Read the model definition and answer for the solid it produces. Units are mm, in the model's axes. A direction names the side the tool comes from. Give positions to 0.01 mm unless a question says otherwise; leave off trailing zeros. Loops run counter-clockwise (first coordinate to the right, second up) from the corner with the lowest first, then second, coordinate; pieces in that order, holes last. Notation, with made-up numbers: M -3,-15 L 4,-15 A33 ccw 4,18 Z; hole C -33,-38 d8. An arc over 180 degrees is marked long. Return JSON: item names as keys, results as strings. Group by question number.
```python
from build123d import *

# Parameters (mm, degrees)
F0_R     = 41.275
F1_DEPTH = 101.6
F2_W     = 82.747999
F2_H     = 29.89918
F3_DEPTH = 36.83
F4_R     = 40.005
F5_DEPTH = 98.044
F6_R     = 41.275
F7_DEPTH = 6.35


with BuildPart() as f1:
    # F0 (on Front) → F1 (new body, symmetric)
    with BuildSketch(Plane.XZ):
        Circle(F0_R)
    extrude(amount=F1_DEPTH, both=True)

    # F2 (on Top) → F3 (cut, symmetric)
    with BuildSketch(Plane.XY):
        with Locations((-0.162097, -78.476146)):
            Rectangle(F2_W, F2_H)
    extrude(amount=F3_DEPTH, both=True, mode=Mode.SUBTRACT)

    # F4 (on Front) → F5 (cut, symmetric)
    with BuildSketch(Plane.XZ):
        Circle(F4_R)
    extrude(amount=F5_DEPTH, both=True, mode=Mode.SUBTRACT)

    # F6 (on face) → F7 (cut, symmetric)
    with BuildSketch(Plane(origin=(0, 101.6, 0), x_dir=(-1, 0, 0), z_dir=(0, 1, 0))):
        Circle(F6_R)
    extrude(amount=F7_DEPTH, both=True, mode=Mode.SUBTRACT)


solid = f1.part
```
1. Straight lines are drawn through the part: line 1 along Z through (x, y) = (0, -51) (3 decimals); line 2 along X through (y, z) = (-54, 0.5); line 3 along Y through (x, z) = (33, 24). For each, find the intervals that lie inside material, in ascending order.
2. Find section B-B (x = -33). Write down the section's boundary in (y, z), and give its area (3 significant figures).
3. Find section D-D (x = 0). Write down the section's boundary in (y, z) (3 decimals).
4. The mould has two halves that part along Y. Classify faces 1 (the flat face through (-1, -101.6, 1)), 2 (the flat face through (-1, -98.044, 1)), 3 (the flat face through (-41, -93.426, 0)): +Y half, -Y half, draft (parallel to the pull), parting line (faces both ways), or undercut.
5. Find section C-C (z = 23.5). Write down the section's boundary in (x, y), and give its area (3 significant figures).
6. Flat-ended cylindrical pins translate along their axes: P1, Ø1.5, axis at y = -34, z = 24.5, coming from the +X side; P2, Ø1.5, axis at y = 72.5, z = 7, coming from the -X side; P3, Ø4, axis at x = -13.5, z = -26, coming from the +Y side. Find the tip coordinate at first contact, or state that the pin passes through.
7. For faces 4 (the cylindrical face through (-39.966, 18.727, 1.759)), 5 (the cylindrical face through (-41.235, 17.319, 1.815)), determine the directions among +Z, -Z, +X, -X, +Y, -Y from which every point of the face is accessible in a straight line to the end or side of a thin tool.
8. Find section A-A (z = 0). Write down the section's boundary in (x, y) (3 decimals), and give its area (3 significant figures).
Result:
{
 "1": {"line 1": "z = -41.275 to -40.005, 40.005 to 41.275", "line 2": "x = -41.27 to -40, 40 to 41.27", "line 3": "y = -101.6 to -93.43, -63.53 to 95.25"},
 "2": {"outline": "M -101.6,-24.79 L -93.43,-24.79 L -93.43,-22.61 L -98.04,-22.61 L -98.04,22.61 L -93.43,22.61 L -93.43,24.79 L -101.6,24.79 Z; M -63.53,-24.79 L 95.25,-24.79 L 95.25,-22.61 L -63.53,-22.61 Z; M -63.53,22.61 L 95.25,22.61 L 95.25,24.79 L -63.53,24.79 Z", "area": "888 mm2"},
 "3": {"outline": "M -101.6,-41.275 L 95.25,-41.275 L 95.25,-40.005 L -98.044,-40.005 L -98.044,40.005 L 95.25,40.005 L 95.25,41.275 L -101.6,41.275 Z"},
 "4": {"face 1": "-Y half", "face 2": "+Y half", "face 3": "undercut"},
 "5": {"outline": "M -33.93,-101.6 L 33.93,-101.6 L 33.93,-93.43 L 32.38,-93.43 L 32.38,-98.04 L -32.38,-98.04 L -32.38,-93.43 L -33.93,-93.43 Z; M -33.93,-63.53 L -32.38,-63.53 L -32.38,95.25 L -33.93,95.25 Z; M 32.38,-63.53 L 33.93,-63.53 L 33.93,95.25 L 32.38,95.25 Z", "area": "750 mm2"},
 "6": {"P1": "stops at x = 33.76", "P2": "stops at x = -40.8", "P3": "stops at y = -98.04"},
 "7": {"face 4": "+Y", "face 5": "+Y, -Y"},
 "8": {"outline": "M -41.275,-101.6 L 41.275,-101.6 L 41.275,95.25 L 40.005,95.25 L 40.005,-63.527 L 41.212,-63.527 L 41.212,-93.426 L 40.005,-93.426 L 40.005,-98.044 L -40.005,-98.044 L -40.005,-93.426 L -41.275,-93.426 Z; M -41.275,-63.527 L -40.005,-63.527 L -40.005,95.25 L -41.275,95.25 Z", "area": "710 mm2"}
}
